Check sheet for the modelled part. Datum: model origin and axes. Units: mm. Face numbers are marked on the shaded views. A direction names the side the tool comes from. Give positions to 0.01 mm unless a question says otherwise; leave off trailing zeros. Loops run counter-clockwise (first coordinate to the right, second up) from the corner with the lowest first, then second, coordinate; pieces in that order, holes last. Notation, with made-up numbers: (18.25, 4.5) - (67.25, 4.5) arc R30 ccw to (67.25, 28.5) - close; hole circle Ø10 at (57, 18.25). An arc over 180 degrees is marked (long way). Answer in a Markdown table with one row per item. Add a question column.
(1) Thickness scan on L1, parallel to X at y = -0.5, z = 1; L2, parallel to Z at x = -1, y = 1.15 (3 decimals); L3, parallel to X at y = 1.4, z = -0.55. Record the ranges inside material, lowest first.
(2) Sectioned sample at D-D on y = -1.45. Enter the section's corners in (x, z) (3 decimals).
(3) Sectioned sample at C-C on x = -2.75. Enter the section's corners in (y, z) (3 decimals).
(4) Go/stop test with a flat-tipped pin: P1, Ø2, axis at x = -3.5, y = 0, coming from the +Z side (3 decimals). Record where the tip stops, or that it passes through.
(5) Set-up check for the marked faces 1 and 2: record each of +Z, -Z, +X, -X, +Y, -Y from which the full face is reachable in a straight line by a thin tool's end or side.
(6) Sectioned sample at A-A on z = 0.9. Enter the section's corners in (x, y) (3 decimals), then the cut area to 3 significant figures.
(7) Sectioned sample at B-B on y = -1. Enter the section's corners in (x, z) (3 decimals).
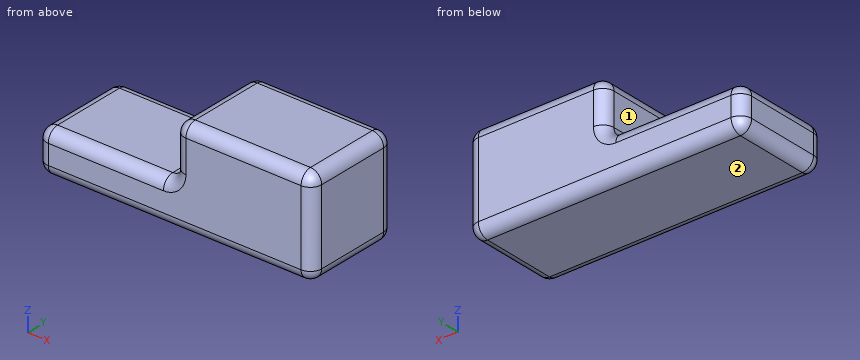
Autodesk Fusion 360 part; units mm, degrees
sketch "Sketch1" plane through (0, 0, 0) normal (1, 0, 0) x (0, 1, 0)
  line L0 (1.725, -1.725) -> (-1.725, -1.725)
  line L1 (-1.725, -1.725) -> (-1.725, 1.725)
  line L2 (-1.725, 1.725) -> (1.725, 1.725)
  line L3 (1.725, 1.725) -> (1.725, -1.725)
  line L4 (1.725, -1.725) -> (-1.725, 1.725) construction
  line L5 (-1.725, -1.725) -> (1.725, 1.725) construction
  line L6 (-1.725, -1.725) -> (1.725, -1.725)
  line L7 (1.725, -1.725) -> (1.725, -0.225)
  line L8 (1.725, -0.225) -> (-1.725, -0.225)
  line L9 (-1.725, -0.225) -> (-1.725, -1.725)
  dimension "d1" = 3.45
  dimension "d2" = 3.45
  dimension "d7" = 1.5
extrude "Extrude1" add sketch "Sketch1" against normal blind 4.9 contours L0 L1 L3 L6 L7 L8 L9
extrude "Extrude3" add sketch "Sketch1" along normal blind 4.9
fillet "Fillet1" radius 0.4 10 edges at (-2.45, -1.725, -0.225) (-2.45, 1.725, -0.225) (0, 0, -0.225) (0, 0, 1.725) (0, -1.725, 0.75) (0, -1.725, -1.725) (2.45, -1.725, 1.725) (2.45, 1.725, 1.725) (0, 1.725, -1.725) (0, 1.725, 0.75) 2 faces at (4.9, -0.575, 0.575) (-4.9, 0.575, -1.225)
equation "d2 = d1"
Reply:
| question | item | result |
|---|---|---|
| 1 | L1 | 0 to 4.9 |
| 1 | L2 | -1.725 to -0.225 |
| 1 | L3 | -4.89 to 4.89 |
| 2 | outline | (-4.88, -1.325) arc R0.38 ccw to (-4.5, -1.705) - (4.5, -1.705) arc R0.38 ccw to (4.88, -1.325) - (4.88, 1.325) arc R0.38 ccw to (4.5, 1.705) - (0.4, 1.705) arc R0.38 ccw to (0.02, 1.325) - (0.02, 0.175) arc R0.42 cw to (-0.4, -0.245) - (-4.5, -0.245) arc R0.38 ccw to (-4.88, -0.625) - close |
| 3 | outline | (-1.725, -1.325) arc R0.4 ccw to (-1.325, -1.725) - (1.325, -1.725) arc R0.4 ccw to (1.725, -1.325) - (1.725, -0.625) arc R0.4 ccw to (1.325, -0.225) - (-1.325, -0.225) arc R0.4 ccw to (-1.725, -0.625) - close |
| 4 | P1 | z = -0.225 |
| 5 | face 1 | +Z, -X, +Y, -Y |
| 5 | face 2 | -Z, +X, -X, +Y, -Y |
| 6 | outline | (0, -1.325) arc R0.4 ccw to (0.4, -1.725) - (4.5, -1.725) arc R0.4 ccw to (4.9, -1.325) - (4.9, 1.325) arc R0.4 ccw to (4.5, 1.725) - (0.4, 1.725) arc R0.4 ccw to (0, 1.325) - close |
| 6 | area | 16.8 mm^2 |
| 7 | outline | (-4.9, -1.325) arc R0.4 ccw to (-4.5, -1.725) - (4.5, -1.725) arc R0.4 ccw to (4.9, -1.325) - (4.9, 1.325) arc R0.4 ccw to (4.5, 1.725) - (0.4, 1.725) arc R0.4 ccw to (0, 1.325) - (0, 0.175) arc R0.4 cw to (-0.4, -0.225) - (-4.5, -0.225) arc R0.4 ccw to (-4.9, -0.625) - close |
